```python
from build123d import *

# Parameters (mm, degrees)
SKETCH051_W  = 300
SKETCH051_H  = 60
PAD_DEPTH    = 150
SKETCH052_W  = 312
SKETCH052_H  = 50
PAD001_DEPTH = 156
SKETCH053_W  = 412
SKETCH053_H  = 412
PAD002_DEPTH = 6


with BuildPart() as body:
    # Sketch051 → Pad (new body, symmetric)
    with BuildSketch(Plane.XZ):
        with Locations((0, 30)):
            Rectangle(SKETCH051_W, SKETCH051_H)
    extrude(amount=PAD_DEPTH, both=True)


with BuildPart() as cut006:
    # Sketch052 → Pad001 (new body, symmetric)
    with BuildSketch(Plane.XZ):
        with Locations((0, 25)):
            Rectangle(SKETCH052_W, SKETCH052_H)
    extrude(amount=PAD001_DEPTH, both=True)

    # Sketch053 (on Face3 of Pad001) → Pad002 (join)
    with BuildSketch(Plane(origin=(0, 0, 50), x_dir=(-1, 0, 0), z_dir=(0, 0, 1))):
        Rectangle(SKETCH053_W, SKETCH053_H)
    extrude(amount=PAD002_DEPTH)

    # Cut006: cut Body
    add(body.part, mode=Mode.SUBTRACT)


solid = cut006.part
```
Part model, mm, in its own coordinate system. A direction names the side the tool comes from. Round coordinates to 2 decimals unless told otherwise and drop trailing zeros. Loops run counter-clockwise (first coordinate to the right, second up) from the corner with the lowest first, then second, coordinate; pieces in that order, holes last.
Item 1: Cut at C-C, the plane z = 31. Give the cut face in (x, y).
Item 2: Cut at A-A, the plane y = -89. Give the cut face in (x, z), then the cut area to 3 significant figures.
Item 3: Drill centre lines: line 1 (Y direction, x = -137, z = 46); line 2 (Z direction, x = 18, y = 179). Where is each one in solid material? Low to high.
Item 4: Drop flat-ended pins along their axis: P1, Ø3, axis at y = -100, z = 49.5, coming from the -X side; P2, Ø10, axis at y = -68.5, z = 42.5, coming from the -X side; P3, Ø17, axis at y = -62, z = 17, coming from the +X side; P4, Ø6, axis at x = 147, z = 34.5, coming from the +Y side. Give the stop position or say it passes through.
Item 5: Mould opens along X. For faces 6 (the face through (-2, -156, 25)), 7 (the face through (-150, -2, 28)), 8 (the face through (-156, -2, 25)) say: +X half, -X half, draft (parallel to the pull), parting line (faces both ways), or undercut.
Item 6: Cut at D-D, the plane y = 166.5. Give the cut face in (x, z).
Item 7: 3-axis set-ups, long thin cutter, end or side, ignore diameter. For faces 1 (the face through (-2, 156, 25)), 2 (the face through (-2, 150, 28)), 3 (the face through (156, -2, 25)), 4 (the face through (-151, -70, 0)), 5 (the face through (-180, -3, 56)): which of +Z, -Z, +X, -X, +Y, -Y reach the whole face in a straight line?
A:
1. outline: (-156, -156) - (156, -156) - (156, 156) - (-156, 156) - close; hole (-150, -150) - (150, -150) - (150, 150) - (-150, 150) - close
2. outline: (-206, 50) - (-156, 50) - (-156, 0) - (-150, 0) - (-150, 56) - (-206, 56) - close; (150, 0) - (156, 0) - (156, 50) - (206, 50) - (206, 56) - (150, 56) - close
2. area: 1,270 mm2
3. line 1: y = -156 to -150, 150 to 156
3. line 2: z = 50 to 56
4. P1: stops at x = -206
4. P2: stops at x = -156
4. P3: stops at x = 156
4. P4: stops at y = 156
5. face 6: draft
5. face 7: undercut
5. face 8: -X half
6. outline: (-206, 50) - (206, 50) - (206, 56) - (-206, 56) - close
7. face 1: -Z, +X, -X, +Y
7. face 2: +Z, -Z
7. face 3: -Z, +X, +Y, -Y
7. face 4: -Z, +X, -X, +Y, -Y
7. face 5: +Z, +X, -X, +Y, -Y
